Geometry: final body of the model. Coordinates: model frame, mm. A direction names the side the tool comes from. Give positions to 0.01 mm unless a question says otherwise; leave off trailing zeros. Write each loop counter-clockwise with the first axis right and the second up, starting at its lowest first coordinate (ties: lowest second). Pieces come first, ordered by that corner, then holes.
Q1. Line query: line 1 (X direction, y = 51, z = -12.5); line 2 (Y direction, x = -15.5, z = -16); line 3 (Z direction, x = -16, y = 8). Output: solid intervals per line, ascending.
Q2. Pin query (flat end, axial travel): pin 1 Ø5 at (x, y) = (-1, 28.5) entering from +Z; pin 2 Ø1.3 at (x, z) = (-29, -29.5) entering from +Y; pin 3 Ø1 at (x, y) = (17.5, 16) entering from +Z. Return the tip coordinate at first contact, or that it passes through.
Q3. Reachability of faces 4 (the flat face through (31.704, 45, -15)), 5 (the flat face through (0, 14, -25.4)), 6 (the flat face through (1, 24, -28.608)), 7 (the cylindrical face through (-0.5, 20.6, -23.5)) from +Z, -Z, +X, -X, +Y, -Y: full face, straight path, thin tool, end or side. Return the list, or none.
Q4. Section A-A (z = -13). Return the cut outline in (x, y).
Q5. Section B-B (y = 41). Return the cut outline in (x, z).
Q6. Section C-C (x = 24). Return the cut outline in (y, z).
Q7. Mould query, pull axis X, two halves, no side actions, for faces 1 (the flat face through (-32.273, 44, -15)), 2 (the flat face through (-12.78, 11.05, -29.4)), 3 (the flat face through (0, 0, 0)). Classes: +X half, -X half, draft (parallel to the pull), parting line (faces both ways), or undercut.
Q8. Section D-D (y = 15). Return the cut outline in (x, z).
from build123d import *

# Parameters (mm, degrees)
SKETCH1_R           = 7.472749452
BOSS_EXTRUDE1_DEPTH = 25.4
SKETCH2_W           = 14.945498904
SKETCH2_H           = 22.418248356
BOSS_EXTRUDE2_DEPTH = 3.20842108
SKETCH4_W           = 63.40856
SKETCH4_H           = 4.26981756
BOSS_EXTRUDE3_DEPTH = 27.00421054
SKETCH6_W           = 27.00421054
SKETCH6_H           = 4.26981756
BOSS_EXTRUDE4_DEPTH = 0.56888896
SKETCH7_W           = 0.56888896
SKETCH7_H           = 27.00421054
BOSS_EXTRUDE5_DEPTH = 38.0746
SKETCH8_W           = 0.56888896
SKETCH8_H           = 27.00421054
BOSS_EXTRUDE6_DEPTH = 0.853447309
SKETCH9_W           = 27.00421054
SKETCH9_H           = 0.853447309
BOSS_EXTRUDE7_DEPTH = 25.37968
BOSS_EXTRUDE8_DEPTH = 3.20842108
FILLET4_R           = 6.35
FILLET5_R           = 6.35
BOSS_EXTRUDE9_DEPTH = 1.60421054


with BuildPart() as part:
    # Sketch1 → Boss-Extrude1 (new body)
    with BuildSketch(Plane.XY):
        Circle(SKETCH1_R)
    extrude(amount=-BOSS_EXTRUDE1_DEPTH)

    # Sketch2 → Boss-Extrude2 (add)
    with BuildSketch(Plane(origin=(0, 0, -25.4), x_dir=(-1, 0, 0), z_dir=(0, 0, -1))):
        with BuildLine():
            ThreePointArc((7.472749452, 0), (0, 7.472749452), (-7.472749452, 0))
            Line((-7.472749452, 0), (7.472749452, 0))
        make_face()
        with BuildLine():
            Line((7.472749452, 0), (-7.472749452, 0))
            ThreePointArc((-7.472749452, 0), (0, -7.472749452), (7.472749452, 0))
        make_face()
        with BuildLine():
            ThreePointArc((7.472749452, 0), (0, 7.472749452), (-7.472749452, 0))
            Line((-7.472749452, 0), (7.472749452, 0))
        make_face()
        with BuildLine():
            Line((7.472749452, 0), (-7.472749452, 0))
            ThreePointArc((-7.472749452, 0), (0, -7.472749452), (7.472749452, 0))
        make_face()
        with Locations((0, 11.209124178)):
            Rectangle(SKETCH2_W, SKETCH2_H)
    extrude(amount=BOSS_EXTRUDE2_DEPTH)

    # Sketch4 → Boss-Extrude3 (add)
    with BuildSketch(Plane(origin=(0, 0, -28.60842108), x_dir=(-1, 0, 0), z_dir=(0, 0, -1))):
        with Locations((0, 24.553157136)):
            Rectangle(SKETCH4_W, SKETCH4_H)
    extrude(amount=-BOSS_EXTRUDE3_DEPTH)

    # Sketch6 → Boss-Extrude4 (add)
    with BuildSketch(Plane(origin=(31.70428, 0, 0), x_dir=(0, 0, -1), z_dir=(1, 0, 0))):
        with Locations((15.10631581, 24.553157136)):
            Rectangle(SKETCH6_W, SKETCH6_H)
    boss_extrude4 = extrude(amount=BOSS_EXTRUDE4_DEPTH)

    # Sketch7 → Boss-Extrude5 (add)
    with BuildSketch(Plane(origin=(0, 26.688065916, 0), x_dir=(1, 0, 0), z_dir=(0, 1, 0))):
        with Locations((31.98872448, 15.10631581)):
            Rectangle(SKETCH7_W, SKETCH7_H)
    boss_extrude5 = extrude(amount=BOSS_EXTRUDE5_DEPTH)

    # Sketch8 → Boss-Extrude6 (add)
    with BuildSketch(Plane(origin=(0, 64.762665916, 0), x_dir=(1, 0, 0), z_dir=(0, 1, 0))):
        with Locations((31.98872448, 15.10631581)):
            Rectangle(SKETCH8_W, SKETCH8_H)
    boss_extrude6 = extrude(amount=BOSS_EXTRUDE6_DEPTH)

    # Sketch9 → Boss-Extrude7 (add)
    with BuildSketch(Plane.ZY.offset(-31.70428)):
        with Locations((-15.10631581, 65.18938957)):
            Rectangle(SKETCH9_W, SKETCH9_H)
    boss_extrude7 = extrude(amount=BOSS_EXTRUDE7_DEPTH)

    # Mirror1: Boss-Extrude4, Boss-Extrude5, Boss-Extrude6, Boss-Extrude7 across plane
    add(boss_extrude4.mirror(Plane(origin=(0, 0, 0), x_dir=(0, 0, 1), z_dir=(1, 0, 0))))
    add(boss_extrude5.mirror(Plane(origin=(0, 0, 0), x_dir=(0, 0, 1), z_dir=(1, 0, 0))))
    add(boss_extrude6.mirror(Plane(origin=(0, 0, 0), x_dir=(0, 0, 1), z_dir=(1, 0, 0))))
    add(boss_extrude7.mirror(Plane(origin=(0, 0, 0), x_dir=(0, 0, 1), z_dir=(1, 0, 0))))

    # Sketch13 → Boss-Extrude8 (add)
    with BuildSketch(Plane(origin=(0, 0, -28.60842108), x_dir=(-1, 0, 0), z_dir=(0, 0, -1))):
        Polygon((-7.472749452, 0), (-32.27316896, 22.418248356), (-7.472749452, 22.418248356), align=None)
        Polygon((7.472749452, 0), (32.27316896, 22.418248356), (7.472749452, 22.418248356), align=None)
    extrude(amount=-BOSS_EXTRUDE8_DEPTH)

    # Fillet4
    fillet4_edges = [part.edges().sort_by_distance(p)[0] for p in [
        (0, 22.418248356, -25.4),
    ]]
    fillet(fillet4_edges, radius=FILLET4_R)

    # Fillet5
    # the kernel refuses this fillet: 6.35 mm, written as the material it adds along each edge
    with BuildSketch(Plane(origin=(0, 0, -25.4), x_dir=(0.003141587485879873, -0.9999950652018582, 0), z_dir=(-0.9999950652018582, -0.003141587485879873, 0))) as fillet5_piece_1_section:
        with BuildLine():
            CenterArc((7.472749452 + FILLET5_R, FILLET5_R), FILLET5_R, 180, 90)
            Line((7.472749452 + FILLET5_R, 0), (7.472749452 + FILLET5_R, -FILLET5_R * 0.02))
            Line((7.472749452 + FILLET5_R, -FILLET5_R * 0.02), (7.472749452 - FILLET5_R * 0.02, -FILLET5_R * 0.02))
            Line((7.472749452 - FILLET5_R * 0.02, -FILLET5_R * 0.02), (7.472749452 - FILLET5_R * 0.02, FILLET5_R))
            Line((7.472749452 - FILLET5_R * 0.02, FILLET5_R), (7.472749452, FILLET5_R))
        make_face()
    fillet5_piece_1 = revolve(axis=Axis((0, 0, -25.4), (0, 0, 1)), revolution_arc=359.64, mode=Mode.PRIVATE)
    fillet5_piece_1 = split(fillet5_piece_1, bisect_by=Plane(origin=(-7.980408712, 0.458896729, -23.585442905), z_dir=(0.6705805717075095, 0.7418367049751783, 0)), keep=Keep.TOP, mode=Mode.PRIVATE)
    fillet5_piece_1 = split(fillet5_piece_1, bisect_by=Plane(origin=(7.980408712, 0.458896729, -23.585442905), z_dir=(-0.6705805717075095, 0.7418367049751783, 0)), keep=Keep.TOP, mode=Mode.PRIVATE)
    add(fillet5_piece_1)
    with BuildSketch(Plane(origin=(7.472749452, 0, -25.4), x_dir=(-0.11463149337271429, -0.9934080836832069, 0), z_dir=(0, 0, -1))) as fillet5_piece_2:
        with BuildLine():
            CenterArc((2.441134842, -6.308141331), FILLET5_R, 96.582370614, 34.723369341)
            Line((-1.750353646, -1.538033968), (-1.834183416, -1.44263182))
            Line((-1.834183416, -1.44263182), (-0.08382977, 0.095402147))
            Line((-0.08382977, 0.095402147), (0.0145582, 0.126162827))
            ThreePointArc((0.0145582, 0.126162827), (0.856612429, 0.077740261), (1.698666659, 0.126162827))
            Line((1.698666659, 0.126162827), (1.713224859, 0))
        make_face()
    extrude(amount=3.20842108)
    with BuildSketch(Plane(origin=(-7.472749452, 0, -25.4), x_dir=(-0.7418367049751787, 0.6705805717075091, 0), z_dir=(0, 0, -1))) as fillet5_piece_3:
        with BuildLine():
            CenterArc((2.330082911, -6.35), FILLET5_R, 90, 34.723369341)
            Line((-1.286971105, -1.1308602), (-1.359312185, -1.026477404))
            ThreePointArc((-1.359312185, -1.026477404), (-0.694800105, -0.507031771), (-0.094213262, 0.085163733))
            Line((-0.094213262, 0.085163733), (0, 0.127))
            Line((0, 0.127), (2.330082911, 0.127))
            Line((2.330082911, 0.127), (2.330082911, 0))
        make_face()
    extrude(amount=3.20842108)
    with BuildSketch(Plane(origin=(7.472749452, 0, -11.419502535), x_dir=(-0.11463149337271447, -0.9934080836832069, 0), z_dir=(0, 0, -1))) as fillet5_piece_4a_section:
        with BuildLine():
            CenterArc((2.441134842, -6.308141331), FILLET5_R, 96.582370614, 34.723369341)
            Line((-1.750353646, -1.538033968), (-1.834183416, -1.44263182))
            Line((-1.834183416, -1.44263182), (-0.08382977, 0.095402147))
            Line((-0.08382977, 0.095402147), (0.0145582, 0.126162827))
            ThreePointArc((0.0145582, 0.126162827), (0.856612429, 0.077740261), (1.698666659, 0.126162827))
            Line((1.698666659, 0.126162827), (1.713224859, 0))
        make_face()
    fillet5_piece_4a = extrude(amount=17.188918545, mode=Mode.PRIVATE)
    fillet5_piece_4a = split(fillet5_piece_4a, bisect_by=Plane(origin=(7.858473842, 0.054386522, -25.4), z_dir=(0, 0, 1)), keep=Keep.TOP, mode=Mode.PRIVATE)
    with BuildSketch(Plane(origin=(0, 0, -25.4), x_dir=(0.003141587485879873, -0.9999950652018582, 0), z_dir=(-0.9999950652018582, -0.003141587485879873, 0))) as fillet5_piece_4b_section:
        with BuildLine():
            CenterArc((7.472749452 + FILLET5_R, FILLET5_R), FILLET5_R, 180, 90)
            Line((7.472749452 + FILLET5_R, 0), (7.472749452 + FILLET5_R, -FILLET5_R * 0.02))
            Line((7.472749452 + FILLET5_R, -FILLET5_R * 0.02), (7.472749452 - FILLET5_R * 0.02, -FILLET5_R * 0.02))
            Line((7.472749452 - FILLET5_R * 0.02, -FILLET5_R * 0.02), (7.472749452 - FILLET5_R * 0.02, FILLET5_R))
            Line((7.472749452 - FILLET5_R * 0.02, FILLET5_R), (7.472749452, FILLET5_R))
        make_face()
    fillet5_piece_4b = revolve(axis=Axis((0, 0, -25.4), (0, 0, 1)), revolution_arc=359.64, mode=Mode.PRIVATE)
    fillet5_piece_4b = split(fillet5_piece_4b, bisect_by=Plane(origin=(2.712448107, -9.20687202, -24.086642783), z_dir=(0.6705805717075095, 0.7418367049751783, 0)), keep=Keep.TOP, mode=Mode.PRIVATE)
    fillet5_piece_4b = split(fillet5_piece_4b, bisect_by=Plane(origin=(4.884392341, -2.339735928, -24.086642783), z_dir=(0.6705805717075095, -0.7418367049751783, 0)), keep=Keep.TOP, mode=Mode.PRIVATE)
    fillet5_piece_4 = fillet5_piece_4a & fillet5_piece_4b
    add(fillet5_piece_4)
    with BuildSketch(Plane(origin=(-7.472749452, 0, -11.419502535), x_dir=(-0.7418367049751784, 0.6705805717075094, 0), z_dir=(0, 0, -1))) as fillet5_piece_5a_section:
        with BuildLine():
            CenterArc((2.330082911, -6.35), FILLET5_R, 90, 34.723369341)
            Line((-1.286971105, -1.1308602), (-1.359312185, -1.026477404))
            ThreePointArc((-1.359312185, -1.026477404), (-0.694800105, -0.507031771), (-0.094213262, 0.085163733))
            Line((-0.094213262, 0.085163733), (0, 0.127))
            Line((0, 0.127), (2.330082911, 0.127))
            Line((2.330082911, 0.127), (2.330082911, 0))
        make_face()
    fillet5_piece_5a = extrude(amount=17.188918545, mode=Mode.PRIVATE)
    fillet5_piece_5a = split(fillet5_piece_5a, bisect_by=Plane(origin=(-7.858473842, 0.054386522, -25.4), z_dir=(0, 0, 1)), keep=Keep.TOP, mode=Mode.PRIVATE)
    with BuildSketch(Plane(origin=(0, 0, -25.4), x_dir=(0.003141587485879873, -0.9999950652018582, 0), z_dir=(-0.9999950652018582, -0.003141587485879873, 0))) as fillet5_piece_5b_section:
        with BuildLine():
            CenterArc((7.472749452 + FILLET5_R, FILLET5_R), FILLET5_R, 180, 90)
            Line((7.472749452 + FILLET5_R, 0), (7.472749452 + FILLET5_R, -FILLET5_R * 0.02))
            Line((7.472749452 + FILLET5_R, -FILLET5_R * 0.02), (7.472749452 - FILLET5_R * 0.02, -FILLET5_R * 0.02))
            Line((7.472749452 - FILLET5_R * 0.02, -FILLET5_R * 0.02), (7.472749452 - FILLET5_R * 0.02, FILLET5_R))
            Line((7.472749452 - FILLET5_R * 0.02, FILLET5_R), (7.472749452, FILLET5_R))
        make_face()
    fillet5_piece_5b = revolve(axis=Axis((0, 0, -25.4), (0, 0, 1)), revolution_arc=359.64, mode=Mode.PRIVATE)
    fillet5_piece_5b = split(fillet5_piece_5b, bisect_by=Plane(origin=(-4.884392341, -2.339735928, -24.086642783), z_dir=(-0.6705805717075095, -0.7418367049751783, 0)), keep=Keep.TOP, mode=Mode.PRIVATE)
    fillet5_piece_5b = split(fillet5_piece_5b, bisect_by=Plane(origin=(-2.712448107, -9.20687202, -24.086642783), z_dir=(-0.6705805717075095, 0.7418367049751783, 0)), keep=Keep.TOP, mode=Mode.PRIVATE)
    fillet5_piece_5 = fillet5_piece_5a & fillet5_piece_5b
    add(fillet5_piece_5)

    # Sketch14 → Boss-Extrude9 (add)
    with BuildSketch(Plane(origin=(0, 0, -28.60842108), x_dir=(-1, 0, 0), z_dir=(0, 0, -1))):
        with BuildLine():
            Line((-32.27316896, 22.418248356), (-25.92316896, 22.418248356))
            Line((-25.92316896, 22.418248356), (0, 0))
            Line((0, 0), (25.92316896, 22.418248356))
            Line((25.92316896, 22.418248356), (32.27316896, 22.418248356))
            Line((32.27316896, 22.418248356), (9.201290481, 1.56250833))
            ThreePointArc((9.201290481, 1.56250833), (7.989618973, 0.077237004), (7.276359928, -1.701931424))
            ThreePointArc((7.276359928, -1.701931424), (0, -7.472749452), (-7.276359928, -1.701931424))
            ThreePointArc((-7.276359928, -1.701931424), (-7.989618973, 0.077237004), (-9.201290481, 1.56250833))
            Line((-9.201290481, 1.56250833), (-32.27316896, 22.418248356))
        make_face()
    extrude(amount=BOSS_EXTRUDE9_DEPTH)


solid = part.part
Computed:
1. line 1: x = -32.27 to -31.7, 31.7 to 32.27
1. line 2: y = 22.42 to 26.69, 64.76 to 65.62
1. line 3: z = -30.21 to -25.4
2. pin 1: stops at z = -1.6
2. pin 2: stops at y = 22.42
2. pin 3: stops at z = -25.39
3. face 4: +Z, -Z
3. face 5: +Z
3. face 6: -Z, +Y
3. face 7: +Z, +X, -X
4. outline: (-32.27, 22.42) - (32.27, 22.42) - (32.27, 65.62) - (6.32, 65.62) - (6.32, 64.76) - (31.7, 64.76) - (31.7, 26.69) - (-31.7, 26.69) - (-31.7, 64.76) - (-6.32, 64.76) - (-6.32, 65.62) - (-32.27, 65.62) - close; circle Ø14.95 at (0, 0)
5. outline: (-32.27, -28.61) - (-31.7, -28.61) - (-31.7, -1.6) - (-32.27, -1.6) - close; (31.7, -28.61) - (32.27, -28.61) - (32.27, -1.6) - (31.7, -1.6) - close
6. outline: (14.94, -30.21) - (20.76, -30.21) - (20.76, -28.61) - (26.69, -28.61) - (26.69, -1.6) - (22.42, -1.6) - (22.42, -19.05) arc R6.35 cw to (16.07, -25.4) - (14.94, -25.4) - close; (64.76, -28.61) - (65.62, -28.61) - (65.62, -1.6) - (64.76, -1.6) - close
7. face 1: -X half
7. face 2: undercut
7. face 3: draft
8. outline: (-24.07, -30.21) - (-17.35, -30.21) - (-17.35, -28.61) - (17.35, -28.61) - (17.35, -30.21) - (24.07, -30.21) - (24.07, -25.4) - (-24.07, -25.4) - close
